Build history of the part. All positions in model axes, mm. A direction names the side the tool comes from. Give positions to 0.01 mm unless a question says otherwise; leave off trailing zeros. Order: outer loops, then holes, each group sorted by start corner. A loop starts at its lowest first (then second) coordinate and runs counter-clockwise, first axis right, second up. Notation, with made-up numbers: (82.5, 87.25) -> (102.5, 87.25) arc R33 cw to (102.5, 116.25) -> close; hole circle Ø11 at (6, -30.5). An arc over 180 degrees is marked (long way). One line per item, written item: value. Start each with the question number.
(1) Probe line 1 (X direction, y = 25, z = 0); line 2 (X direction, y = 9, z = 3); line 3 (Y direction, x = -13.6, z = 0) (3 decimals). List the from-to ranges inside material, lowest first.
(2) Saw through at A-A on x = 0. Give the cut face in (y, z).
(3) Saw through at C-C on x = 9. Give the cut face in (y, z) (3 decimals), plus the area to 3 significant figures.
(4) Saw through at D-D on z = 5.5. Give the cut face in (x, y).
(5) Pin check, flat tips, straight feed: pin 1 (8 mm diameter, centred on x = 1, z = 3, fed in from +Y); pin 2 (3 mm diameter, centred on y = 38.5, z = -1.5, fed in from -X); pin 3 (12 mm diameter, centred on x = 10.5, y = 14, fed in from -Z). Stop position of each tip, or through.
(6) Which spindle directions (+Z, -Z, +X, -X, +Y, -Y) get a long thin tool onto all of the face, cutting with end or side? Do faces 1 (the flat face through (-5.08, 40, 3)), 2 (the cylindrical face through (-13.275, 2.263, -1.465)), 3 (the cylindrical face through (0, 5.2, -12.7)). Say none if no direction does.
(7) Saw through at B-B on y = 5.08. Give the cut face in (x, z) (3 decimals).
(8) Two-plate mould, pull along X, no slides. Class faces 4 (the cylindrical face through (5.04, 1.98, 0.69)), 5 (the flat face through (0, 10.16, -8)), 6 (the flat face through (2.54, 9, 0)): +X half, -X half, draft (parallel to the pull), parting line (faces both ways), or undercut.
```python
from build123d import *

# Parameters (mm, degrees)
SKETCH1_R               = 14.224
BOSS_EXTRUDE1_DEPTH     = 45.3136
CUT_EXTRUDE1_DEPTH      = 10.16
CUT_EXTRUDE2_START      = -10.16
CUT_EXTRUDE2_DEPTH      = 10.16
CUT_EXTRUDE3_DEPTH      = 52.266840521
CUT_EXTRUDE3_DEPTH_BACK = 52.266840521
SKETCH4_R               = 3.175
SKETCH5_R               = 2.54
CUT_EXTRUDE4_DEPTH      = 41.502098192


with BuildPart() as part:
    # Sketch1 → Boss-Extrude1 (new body)
    with BuildSketch(Plane(origin=(0, 0, 0), x_dir=(1, 0, 0), z_dir=(0, 1, 0))):
        with Locations(Location((0, 0, 0), (0, 0, 90))):
            Circle(SKETCH1_R)
    extrude(amount=BOSS_EXTRUDE1_DEPTH)

    # Sketch2 → Cut-Extrude1 (cut)
    with BuildSketch(Plane(origin=(0, 45.3136, 0), x_dir=(1, 0, 0), z_dir=(0, 1, 0))):
        with BuildLine():
            Line((5.08, 11.639742265), (5.08, -11.639742265))
            ThreePointArc((5.08, -11.639742265), (0, -12.7), (-5.08, -11.639742265))
            Line((-5.08, -11.639742265), (-5.08, 11.639742265))
            ThreePointArc((-5.08, 11.639742265), (0, 12.7), (5.08, 11.639742265))
        make_face()
    extrude(amount=-CUT_EXTRUDE1_DEPTH, mode=Mode.SUBTRACT)

    # Sketch3 → Cut-Extrude2 (cut)
    with BuildSketch(Plane.XZ.offset(CUT_EXTRUDE2_START)):
        with BuildLine():
            Line((-2.54, 12.443407893), (-2.54, -12.443407893))
            ThreePointArc((-2.54, -12.443407893), (0, -12.7), (2.54, -12.443407893))
            Line((2.54, -12.443407893), (2.54, 12.443407893))
            ThreePointArc((2.54, 12.443407893), (0, 12.7), (-2.54, 12.443407893))
        make_face()
        with BuildLine():
            Line((-7.62, 10.16), (-7.62, -10.16))
            ThreePointArc((-7.62, -10.16), (-12.7, 0), (-7.62, 10.16))
        make_face()
        with BuildLine():
            Line((7.62, 10.16), (7.62, -10.16))
            ThreePointArc((7.62, -10.16), (12.7, 0), (7.62, 10.16))
        make_face()
    extrude(amount=CUT_EXTRUDE2_DEPTH, mode=Mode.SUBTRACT)

    # Sketch4 → Cut-Extrude3 (cut, two sides: drawn at the far end of the back side and taken through both)
    with BuildSketch(Plane(origin=(-5.08, 0, 0), x_dir=(0, 0, -1), z_dir=(1, 0, 0)).offset(-CUT_EXTRUDE3_DEPTH_BACK)):
        with Locations((1.060257735, 40.2336)):
            Circle(SKETCH4_R)
        with Locations((0, 5.08)):
            Circle(SKETCH4_R)
    extrude(amount=CUT_EXTRUDE3_DEPTH + CUT_EXTRUDE3_DEPTH_BACK, mode=Mode.SUBTRACT)

    # Sketch5 → Cut-Extrude4 (cut, through all)
    with BuildSketch(Plane(origin=(0, 35.1536, 0), x_dir=(1, 0, 0), z_dir=(0, 1, 0))):
        with Locations(Location((0, 0, 0), (0, 0, 270))):
            Circle(SKETCH5_R)
    extrude(amount=-CUT_EXTRUDE4_DEPTH, mode=Mode.SUBTRACT)


solid = part.part
```
Results below:
1. line 1: x = -14.22 to -2.54, 2.54 to 14.22
1. line 2: x = -13.9 to -12.34, -7.62 to -2.54, 2.54 to 7.62, 12.34 to 13.9
1. line 3: y = 0 to 1.905, 8.255 to 37.241, 43.226 to 45.314
2. outline: (0, -14.22) -> (45.31, -14.22) -> (45.31, -12.7) -> (35.15, -12.7) -> (35.15, -2.54) -> (10.16, -2.54) -> (10.16, -12.7) -> (0, -12.7) -> close; (0, 12.7) -> (10.16, 12.7) -> (10.16, 2.54) -> (35.15, 2.54) -> (35.15, 12.7) -> (45.31, 12.7) -> (45.31, 14.22) -> (0, 14.22) -> close
3. outline: (0, -11.015) -> (45.314, -11.015) -> (45.314, 11.015) -> (0, 11.015) -> (0, 8.96) -> (10.16, 8.96) -> (10.16, -8.96) -> (0, -8.96) -> close; hole circle Ø6.35 at (40.234, -1.06)
3. area: 784 mm²
4. outline: (-13.12, 0) -> (-11.45, 0) -> (-11.45, 10.16) -> (-7.62, 10.16) -> (-7.62, 0) -> (-2.54, 0) -> (-2.54, 10.16) -> (2.54, 10.16) -> (2.54, 0) -> (7.62, 0) -> (7.62, 10.16) -> (11.45, 10.16) -> (11.45, 0) -> (13.12, 0) -> (13.12, 45.31) -> (5.08, 45.31) -> (5.08, 35.15) -> (-5.08, 35.15) -> (-5.08, 45.31) -> (-13.12, 45.31) -> close
5. pin 1: stops at y = 35.15
5. pin 2: stops at x = -14.18
5. pin 3: stops at z = -13.49
6. face 1: +Y
6. face 2: +X, -X
6. face 3: -Y
7. outline: (-13.865, -3.175) arc R14.224 ccw to (13.865, -3.175) -> (12.297, -3.175) arc R12.7 cw to (7.62, -10.16) -> (7.62, -3.175) -> (2.54, -3.175) -> (2.54, -12.443) arc R12.7 cw to (-2.54, -12.443) -> (-2.54, -3.175) -> (-7.62, -3.175) -> (-7.62, -10.16) arc R12.7 cw to (-12.297, -3.175) -> close; (-13.865, 3.175) -> (-12.297, 3.175) arc R12.7 cw to (-7.62, 10.16) -> (-7.62, 3.175) -> (-2.54, 3.175) -> (-2.54, 12.443) arc R12.7 cw to (2.54, 12.443) -> (2.54, 3.175) -> (7.62, 3.175) -> (7.62, 10.16) arc R12.7 cw to (12.297, 3.175) -> (13.865, 3.175) arc R14.224 ccw to start
8. face 4: draft
8. face 5: undercut
8. face 6: undercut
